```python
from build123d import *

# Parameters (mm, degrees)
SKETCH1_R           = 10
BOSS_EXTRUDE1_DEPTH = 90
SKETCH2_W           = 32
SKETCH2_H           = 20
CUT_EXTRUDE1_DEPTH  = 30
FILLET1_R           = 3
CUT_EXTRUDE2_DEPTH  = 55
SKETCH6_W           = 93.565518088
SKETCH6_H           = 91.977475816
CUT_EXTRUDE3_DEPTH  = 55


with BuildPart() as part:
    # Sketch1 → Boss-Extrude1 (new body)
    with BuildSketch(Plane.XY):
        with BuildLine():
            Line((-30, 12.5), (-18, 12.5))
            Line((-18, 12.5), (-18, 22.5))
            Line((-18, 22.5), (-12, 22.5))
            Line((-12, 22.5), (-12, 57.5))
            Line((-12, 57.5), (12, 57.5))
            Line((12, 57.5), (12, 22.5))
            Line((12, 22.5), (18, 22.5))
            Line((18, 22.5), (18, 12.5))
            Line((18, 12.5), (30, 12.5))
            ThreePointArc((30, 12.5), (42.5, 0), (30, -12.5))
            Line((30, -12.5), (-30, -12.5))
            ThreePointArc((-30, -12.5), (-42.5, 0), (-30, 12.5))
        make_face()
        with Locations((0, 12.5)):
            Circle(SKETCH1_R, mode=Mode.SUBTRACT)
    extrude(amount=-BOSS_EXTRUDE1_DEPTH)

    # Sketch2 → Cut-Extrude1 (cut)
    with BuildSketch(Plane(origin=(12, 0, 0), x_dir=(0, 0, -1), z_dir=(1, 0, 0))):
        with Locations((74, 47.5)):
            Rectangle(SKETCH2_W, SKETCH2_H)
    extrude(amount=-CUT_EXTRUDE1_DEPTH, mode=Mode.SUBTRACT)

    # Fillet1
    fillet1_edges = [part.edges().sort_by_distance(p)[0] for p in [
        (0, 37.5, -58),
    ]]
    fillet(fillet1_edges, radius=FILLET1_R)

    # Sketch3 → Cut-Extrude2 (cut)
    with BuildSketch(Plane.XY):
        Polygon((0, 47.5), (-6, 32.5), (6, 32.5), align=None)
    extrude(amount=-CUT_EXTRUDE2_DEPTH, mode=Mode.SUBTRACT)

    # Sketch6 → Cut-Extrude3 (cut)
    with BuildSketch(Plane(origin=(0, -3.125, -5.412658774), x_dir=(1, 0, 0), z_dir=(0, 0.5, 0.866025404))):
        with Locations((1.570824933, 32.896964302)):
            Rectangle(SKETCH6_W, SKETCH6_H)
    extrude(amount=CUT_EXTRUDE3_DEPTH, mode=Mode.SUBTRACT)


solid = part.part
```
For this review, take the finished solid that the model builds, in its own axes (mm). A direction names the side the tool comes from. Round coordinates to 2 decimals unless told otherwise and drop trailing zeros. Write each loop counter-clockwise with the first axis right and the second up, starting at its lowest first coordinate (ties: lowest second). Pieces come first, ordered by that corner, then holes.
1) For line 1 along Y through (x, z) = (0, -61.5); line 2 along Y through (x, z) = (0, -30); line 3 along Y through (x, z) = (-13, -83.5), list the stretches that pass through material, from the lowest coordinate up.
Answer below:
line 1: y = -12.5 to 2.5, 22.5 to 37.5
line 2: y = -12.5 to 2.5, 22.5 to 32.5
line 3: y = -12.5 to 22.5
2) Take a section at B-B on y = 15.5. Give the boundary of the cut face in (x, z), then the cut area to 3 significant figures.
Answer below:
outline: (-18, -90) - (-9.54, -90) - (-9.54, -16.17) - (-18, -16.17) - close; (9.54, -90) - (18, -90) - (18, -16.17) - (9.54, -16.17) - close
area: 1,250 mm2
3) Take a section at D-D on y = 43. Give the boundary of the cut face in (x, z), then the cut area to 3 significant figures.
Answer below:
outline: (-12, -58) - (12, -58) - (12, -32.04) - (1.8, -32.04) - (1.8, -55) - (-1.8, -55) - (-1.8, -32.04) - (-12, -32.04) - close
area: 540 mm2
4) Insertion check: pin 1 Ø12 at (y, z) = (3.5, -55) entering from +X; pin 2 Ø6 at (x, z) = (-25, -40.5) entering from +Y; pin 3 Ø17.5 at (y, z) = (48, -50) entering from +X; pin 4 Ø3.5 at (x, z) = (-3, -38.5) entering from +Y. Each pin has a flat end and moves straight along its axis. Give the tip position at first contact, or say it passes through.
Answer below:
pin 1: stops at x = 42.5
pin 2: stops at y = 12.5
pin 3: stops at x = 12
pin 4: stops at y = 57.22
5) Mouldability with a two-part tool opening along X and no side actions: class faces 1 (the face through (-42.497, -0.275, -44.37)), 2 (the face through (0, 32.5, -40)), 3 (the face through (-3, 40, -44)), 4 (the face through (0, 57.5, -49)) as +X half, -X half, draft (parallel to the pull), parting line (faces both ways), or undercut.
Answer below:
face 1: -X half
face 2: undercut
face 3: undercut
face 4: draft
6) Take a section at C-C on z = -30. Give the boundary of the cut face in (x, y).
Answer below:
outline: (-30, -12.5) - (30, -12.5) arc R12.5 ccw to (30, 12.5) - (18, 12.5) - (18, 22.5) - (12, 22.5) - (12, 39.46) - (3.22, 39.46) - (6, 32.5) - (-6, 32.5) - (-3.22, 39.46) - (-12, 39.46) - (-12, 22.5) - (-18, 22.5) - (-18, 12.5) - (-30, 12.5) arc R12.5 ccw to start; hole circle Ø20 at (0, 12.5)
7) Machinability: for faces 5 (the face through (3, 40, -44)), 6 (the face through (-15, 22.5, -55)), 7 (the face through (0, 37.5, -75)), 8 (the face through (15, 22.5, -55)), which of the approach directions +Z, -Z, +X, -X, +Y, -Y give a long, thin tool a straight path to every point of the face, cutting with its end or side? Answer none if there is none.
Answer below:
face 5: +Z
face 6: +Z, -Z, -X, +Y
face 7: -Z, +X, -X, +Y
face 8: +Z, -Z, +X, +Y
8) Take a section at A-A on x = 2. Give the boundary of the cut face in (y, z).
Answer below:
outline: (-12.5, -90) - (2.7, -90) - (2.7, -8.78) - (-12.5, 0) - close; (22.3, -90) - (37.5, -90) - (37.5, -61) arc R3 cw to (40.5, -58) - (57.5, -58) - (57.5, -40.41) - (42.5, -31.75) - (42.5, -55) - (32.5, -55) - (32.5, -25.98) - (22.3, -20.09) - close
